Can you work these out from the model? Positions are in its coordinate system, mm. Face numbers are marked on the shaded views. A direction names the side the tool comes from. Give positions to 0.01 mm unless a question says otherwise; leave off trailing zeros. Write each loop counter-clockwise with the first axis right and the second up, starting at its lowest first coordinate (ties: lowest second). Pieces come first, ordered by that corner, then holes. Notation, with made-up numbers: (47, 86.5) -> (62, 86.5) arc R19 cw to (62, 109.5) -> close; hole circle Ø3 at (4.25, -16.75). An arc over 180 degrees is marked (long way). Answer as CSV lines item,"result". Start each with the question number.
1. On a 3-axis mill with a long thin cutter (end or side, diameter ignored), from which of +Z, -Z, +X, -X, +Y, -Y can I reach the whole of each face in a straight line? I mean the marked faces 1 and 2. Say none if no direction works.
2. I need wall thicknesses on line 1 (X direction, y = -2.2, z = 0.8); line 2 (Y direction, x = 1, z = 1.2); line 3 (X direction, y = 0.2, z = 1.05). Which ranges of each line are inside material? Lowest first, please. Write a range as [from, to].
3. I'm going to push a flat-ended pin straight in: P1, Ø3, axis at x = -0.5, y = 1.5, coming from the -Z side. Where does the tip first touch, or does it pass through?
4. If we section it at C-C on z = 1.2: Write out the boundary of the cut face in (x, y), plus the area to 3 significant figures.
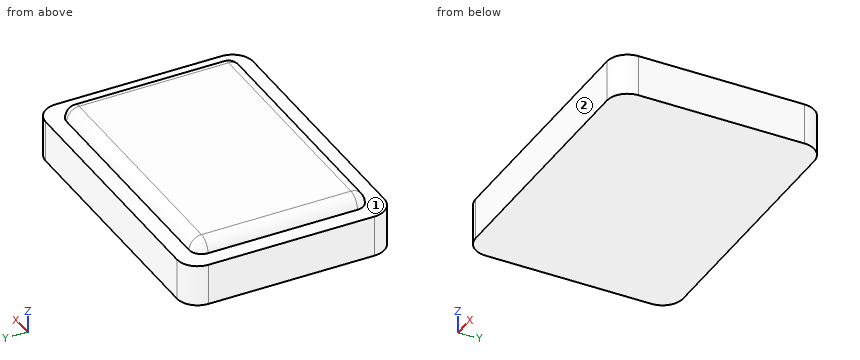
```python
from build123d import *

# Parameters (mm, degrees)
SKETCH_1_W      = 7
SKETCH_1_H      = 5
EXTRUDE_1_DEPTH = 1
FILLET_1_R      = 0.5
SKETCH_2_W      = 6.2
SKETCH_2_H      = 4.2
EXTRUDE_2_DEPTH = 0.3
FILLET_2_R      = 0.3


with BuildPart() as part:
    # Эскиз1 → Бобышка-Вытянуть1 (new body)
    with BuildSketch(Plane.XY):
        Rectangle(SKETCH_1_W, SKETCH_1_H)
    extrude(amount=EXTRUDE_1_DEPTH)

    # Скругление1
    fillet_1_edges = [part.edges().sort_by_distance(p)[0] for p in [
        (3.5, -2.5, 0.5),
        (-3.5, -2.5, 0.5),
        (-3.5, 2.5, 0.5),
        (3.5, 2.5, 0.5),
    ]]
    fillet(fillet_1_edges, radius=FILLET_1_R)

    # Эскиз2 → Бобышка-Вытянуть2 (add)
    with BuildSketch(Plane.XY.offset(1)):
        Rectangle(SKETCH_2_W, SKETCH_2_H)
    extrude(amount=EXTRUDE_2_DEPTH)

    # Скругление2
    fillet_2_edges = [part.edges().sort_by_distance(p)[0] for p in [
        (3.1, -2.1, 1.15),
        (3.1, 2.1, 1.15),
        (-3.1, 2.1, 1.15),
        (-3.1, -2.1, 1.15),
        (3.1, 0, 1.3),
        (0, 2.1, 1.3),
        (-3.1, 0, 1.3),
        (0, -2.1, 1.3),
    ]]
    fillet(fillet_2_edges, radius=FILLET_2_R - 0.0001)  # a hair under: the kernel refuses the full size


solid = part.part
```
Computed values:
1,face 1,"+Z"
1,face 2,"+Z, -Z, +X, -X, -Y"
2,line 1,"x = [-3.46, 3.46]"
2,line 2,"y = [-2.02, 2.02]"
2,line 3,"x = [-3.1, 3.1]"
3,P1,"stops at z = 0"
4,outline,"(-3.02, -1.8) arc R0.22 ccw to (-2.8, -2.02) -> (2.8, -2.02) arc R0.22 ccw to (3.02, -1.8) -> (3.02, 1.8) arc R0.22 ccw to (2.8, 2.02) -> (-2.8, 2.02) arc R0.22 ccw to (-3.02, 1.8) -> close"
4,area,"24.4 mm2"
